Verification items for the finished model (mm, model axes). A direction names the side the tool comes from. Give positions to 0.01 mm unless a question says otherwise; leave off trailing zeros. Write each loop counter-clockwise with the first axis right and the second up, starting at its lowest first coordinate (ties: lowest second). Pieces come first, ordered by that corner, then holes. Notation, with made-up numbers: M 76.5,47 L 104.5,47 A15 ccw 104.5,58 Z; hole C -16.5,-18.75 d10. An arc over 180 degrees is marked long. Answer as a JSON object with one key per item and string values.
```python
from build123d import *

# Parameters (mm, degrees)
HUB_START   = 2.2
SKETCH1_R   = 7
SKETCH1_R_2 = 3.05
HUB_DEPTH   = 4.3
ARM_START   = 6.5
SKETCH2_R   = 1.6
SKETCH2_R_2 = 0.8
ARM_DEPTH   = 2.5


with BuildPart() as part:
    # Sketch1 → Hub (new body)
    with BuildSketch(Plane.XY.offset(HUB_START)):
        with Locations(Location((0, 0, 0), (0, 0, 180))):
            Circle(SKETCH1_R)
        with Locations(Location((0, 0, 0), (0, 0, 180))):
            Circle(SKETCH1_R_2, mode=Mode.SUBTRACT)
    extrude(amount=HUB_DEPTH)

    # Sketch2 → Arm (add)
    with BuildSketch(Plane.XY.offset(ARM_START)):
        with BuildLine():
            Line((-11, 4), (11, 4))
            ThreePointArc((11, 4), (15, 0), (11, -4))
            Line((11, -4), (-11, -4))
            ThreePointArc((-11, -4), (-15, 0), (-11, 4))
        make_face()
        Circle(SKETCH2_R, mode=Mode.SUBTRACT)
        with Locations((-10, 0)):
            Circle(SKETCH2_R_2, mode=Mode.SUBTRACT)
        with Locations((10, 0)):
            Circle(SKETCH2_R_2, mode=Mode.SUBTRACT)
    extrude(amount=ARM_DEPTH)


solid = part.part
```
1) Section check A-A on x = 0. Record the boundary of the cut face in (y, z).
Completed:
{"outline": "M -7,2.2 L -3.05,2.2 L -3.05,6.5 L -1.6,6.5 L -1.6,9 L -4,9 L -4,6.5 L -7,6.5 Z; M 1.6,6.5 L 3.05,6.5 L 3.05,2.2 L 7,2.2 L 7,6.5 L 4,6.5 L 4,9 L 1.6,9 Z"}
2) Section check B-B on y = 0. Record the boundary of the cut face in (x, z), and give its area (3 significant figures).
Completed:
{"outline": "M -15,6.5 L -10.8,6.5 L -10.8,9 L -15,9 Z; M -9.2,6.5 L -7,6.5 L -7,2.2 L -3.05,2.2 L -3.05,6.5 L -1.6,6.5 L -1.6,9 L -9.2,9 Z; M 1.6,6.5 L 3.05,6.5 L 3.05,2.2 L 7,2.2 L 7,6.5 L 9.2,6.5 L 9.2,9 L 1.6,9 Z; M 10.8,6.5 L 15,6.5 L 15,9 L 10.8,9 Z", "area": "93.0 mm2"}
3) Access from +Z, -Z, +X, -X, +Y, -Y to the whole of each face (thin tool, end or side, straight path). Record for faces 5 (the face through (0, -5, 6.5)), 6 (the face through (9.41, 0.54, 7.73)), 7 (the face through (3.047, -0.134, 4.32)).
Completed:
{"face 5": "+Z, +X, -X, -Y", "face 6": "+Z, -Z", "face 7": "-Z"}
4) Go/stop test with flat-tipped pins: pin 1 (0.9 mm diameter, centred on x = -2, y = 5.5, fed in from +Z); pin 2 (4 mm diameter, centred on x = -10.5, y = 1, fed in from -Z); pin 3 (0.8 mm diameter, centred on x = -5, z = 8, fed in from -Y). Record where each tip stops, or that it passes through.
Completed:
{"pin 1": "stops at z = 6.5", "pin 2": "stops at z = 6.5", "pin 3": "stops at y = -4"}
5) Section check C-C on z = 7.5. Record the boundary of the cut face in (x, y).
Completed:
{"outline": "M -11,-4 L 11,-4 A4 ccw 11,4 L -11,4 A4 ccw Z; hole C -10,0 d1.6; hole C 0,0 d3.2; hole C 10,0 d1.6"}
6) Thickness scan on L1, parallel to Y at x = 10, z = 7.1; L2, parallel to Y at x = 0, z = 7.45; L3, parallel to Z at x = 13, y = -2.25. Record the ranges inside material, lowest first.
Completed:
{"L1": "y = -4 to -0.8, 0.8 to 4", "L2": "y = -4 to -1.6, 1.6 to 4", "L3": "z = 6.5 to 9"}
7) Release check for a two-part mould opening along Y. For faces 1 (the face through (0, 4, 8)), 2 (the face through (0, 5, 6.5)), 3 (the face through (-1.27, -0.97, 7.73)), 4 (the face through (-1.3, -1.3, 6.5)) record: pulls with the +Y half, pulls with the -Y half, needs draft (parallel to the pull), parting line crosses it, or undercut.
Completed:
{"face 1": "pulls with the +Y half", "face 2": "needs draft", "face 3": "undercut", "face 4": "undercut"}
8) Section check D-D on x = -10. Record the boundary of the cut face in (y, z).
Completed:
{"outline": "M -4,6.5 L -0.8,6.5 L -0.8,9 L -4,9 Z; M 0.8,6.5 L 4,6.5 L 4,9 L 0.8,9 Z"}
